from build123d import *

# Parameters (mm, degrees)
SKETCH1_W                  = 44.45
SKETCH1_H                  = 60
CUT_EXTRUDE1_START         = -50
CUT_EXTRUDE1_DEPTH         = 50
M4X0_7_TAPPED_HOLE1_D      = 3.3
M4X0_7_TAPPED_HOLE1_DEPTH  = 10
M4X0_7_TAPPED_HOLE1_TIP    = 0.991420021
M3X0_5_TAPPED_HOLE1_REACH  = 117.544
M3X0_5_TAPPED_HOLE1_BORE_R = 1.25
M3X0_5_TAPPED_HOLE2_REACH  = 117.544
M3X0_5_TAPPED_HOLE2_BORE_R = 1.25


with BuildPart() as part:
    # Sketch1 → Revolve1 (revolve)
    with BuildSketch(Plane.XZ, mode=Mode.PRIVATE) as revolve1_sk:
        with Locations((22.225, 30)):
            Rectangle(SKETCH1_W, SKETCH1_H)
    revolve(revolve1_sk.sketch.rotate(Axis((0, 0, 60), (0, 0, -1)), 180), axis=Axis((0, 0, 60), (0, 0, -1)))

    # Sketch2 → Cut-Extrude1 (cut)
    with BuildSketch(Plane(origin=(0, 0, 0), x_dir=(-1, 0, 0), z_dir=(0, 0, -1)).offset(CUT_EXTRUDE1_START)):
        with BuildLine():
            Line((43.7241638, 8), (43.7241638, -8))
            ThreePointArc((43.7241638, -8), (44.45, 0), (43.7241638, 8))
        make_face()
    extrude(amount=CUT_EXTRUDE1_DEPTH, mode=Mode.SUBTRACT)

    # Sketch3 → Cut-Revolve1 (revolve, cut)
    with BuildSketch(Plane.XZ, mode=Mode.PRIVATE) as cut_revolve1_sk:
        Polygon((37.5, 60), (0, 60), (0, 0), (37.5, 0), (37.5, 20.5), (32, 20.5), (32, 39.5), (37.5, 39.5), align=None)
    revolve(cut_revolve1_sk.sketch.rotate(Axis((0, 0, 60), (0, 0, -1)), 180), axis=Axis((0, 0, 60), (0, 0, -1)), mode=Mode.SUBTRACT)

    # M4x0.7 Tapped Hole1
    with Locations(Plane.XY.offset(60)):
        with Locations((28.991378029, 28.991378029), (0, 41), (-28.991378029, 28.991378029), (-41, 0), (-28.991378029, -28.991378029), (0, -41), (28.991378029, -28.991378029), (41, 0)):
            Hole(M4X0_7_TAPPED_HOLE1_D / 2, depth=M4X0_7_TAPPED_HOLE1_DEPTH)
            with Locations((0, 0, -(M4X0_7_TAPPED_HOLE1_DEPTH + M4X0_7_TAPPED_HOLE1_TIP / 2))):  # 118° drill point
                Cone(0, M4X0_7_TAPPED_HOLE1_D / 2, M4X0_7_TAPPED_HOLE1_TIP, mode=Mode.SUBTRACT)

    # M3x0.5 Tapped Hole1 bore → M3x0.5 Tapped Hole1 (cut, up to next)
    with BuildSketch(Plane.ZY.offset(43.7241638), mode=Mode.PRIVATE) as m3x0_5_tapped_hole1_sk1:
        with Locations((15.584748033, 5.15)):
            Circle(M3X0_5_TAPPED_HOLE1_BORE_R)
    m3x0_5_tapped_hole1_tool1 = extrude(m3x0_5_tapped_hole1_sk1.sketch, amount=-M3X0_5_TAPPED_HOLE1_REACH, mode=Mode.PRIVATE) & part.part
    add(m3x0_5_tapped_hole1_tool1.solids().sort_by_distance((-43.724164, 5.15, 15.584748))[0], mode=Mode.SUBTRACT)

    # M3x0.5 Tapped Hole2 bore → M3x0.5 Tapped Hole2 (cut, up to next)
    with BuildSketch(Plane.ZY.offset(43.7241638), mode=Mode.PRIVATE) as m3x0_5_tapped_hole2_sk1:
        with Locations((37.834748033, -5.05)):
            Circle(M3X0_5_TAPPED_HOLE2_BORE_R)
    m3x0_5_tapped_hole2_tool1 = extrude(m3x0_5_tapped_hole2_sk1.sketch, amount=-M3X0_5_TAPPED_HOLE2_REACH, mode=Mode.PRIVATE) & part.part
    add(m3x0_5_tapped_hole2_tool1.solids().sort_by_distance((-43.724164, -5.05, 37.834748))[0], mode=Mode.SUBTRACT)


solid = part.part
CAD build for the part. Positions are in the model's coordinates, mm. A direction names the side the tool comes from. Give positions to 0.01 mm unless a question says otherwise; leave off trailing zeros. Write each loop counter-clockwise with the first axis right and the second up, starting at its lowest first coordinate (ties: lowest second). Pieces come first, ordered by that corner, then holes. Notation, with made-up numbers: (68.25, -21.75) -> (87.25, -21.75) arc R21 cw to (87.25, -13.75) -> close; hole circle Ø1 at (40.25, 67.5). An arc over 180 degrees is marked (long way). Return JSON: item names as keys, results as strings.
Item 1: Band-saw the part on C-C (z = 54). Give the number of separate pieces and of enclosed holes in the cut face, then the cut area to 3 significant figures.
Answer below:
{"separate pieces": "1", "enclosed holes": "9", "area": "1,720 mm2"}
Item 2: Two-plate mould, pull along X, no slides. Class faces 5 (the cylindrical face through (-41.061, -17.025, 30.42)), 6 (the flat face through (28, 17, 39.5)), 7 (the flat face through (-32, -20, 0)): +X half, -X half, draft (parallel to the pull), parting line (faces both ways), or undercut.
Answer below:
{"face 5": "parting line", "face 6": "undercut", "face 7": "draft"}
Item 3: Tool access for faces 1 (the cylindrical face through (-37.635, -4.995, 36.586)), 2 (the cylindrical face through (42.65, 0.07, 54.93)), 3 (the flat face through (-43.724, 0, 25)), 4 (the cylindrical face through (-17.3, -33.27, 10.39)): list every direction of +Z, -Z, +X, -X, +Y, -Y with a clear straight run to the whole face (end or side of a thin tool).
Answer below:
{"face 1": "-X", "face 2": "+Z", "face 3": "-Z, -X, +Y, -Y", "face 4": "-Z"}
Item 4: Drop flat-ended pins along their axis: pin 1 (4 mm diameter, centred on x = 26.5, z = 23, fed in from +Y); pin 2 (2 mm diameter, centred on y = -5.05, z = 37.83, fed in from +X); pin 3 (12 mm diameter, centred on y = 10, z = 30, fed in from -X). Give the stop position or say it passes through.
Answer below:
{"pin 1": "stops at y = 37.09", "pin 2": "stops at x = 44.27", "pin 3": "stops at x = -43.72"}
Item 5: Band-saw the part on B-B (y = 5.15). List the corners of the cut face in (x, z), then the cut area to 3 significant figures.
Answer below:
{"outline": "(-44.15, 50) -> (-43.72, 50) -> (-43.72, 16.83) -> (-37.14, 16.83) -> (-37.14, 20.5) -> (-31.58, 20.5) -> (-31.58, 39.5) -> (-37.14, 39.5) -> (-37.14, 60) -> (-44.15, 60) -> close; (-43.72, 0) -> (-37.14, 0) -> (-37.14, 14.33) -> (-43.72, 14.33) -> close; (31.58, 20.5) -> (37.14, 20.5) -> (37.14, 0) -> (44.15, 0) -> (44.15, 60) -> (37.14, 60) -> (37.14, 39.5) -> (31.58, 39.5) -> close", "area": "1,010 mm2"}
Item 6: Band-saw the part on A-A (x = -3). List the corners of the cut face in (y, z).
Answer below:
{"outline": "(-44.35, 0) -> (-37.38, 0) -> (-37.38, 20.5) -> (-31.86, 20.5) -> (-31.86, 39.5) -> (-37.38, 39.5) -> (-37.38, 60) -> (-44.35, 60) -> close; (31.86, 20.5) -> (37.38, 20.5) -> (37.38, 0) -> (44.35, 0) -> (44.35, 60) -> (37.38, 60) -> (37.38, 39.5) -> (31.86, 39.5) -> close"}
Item 7: Band-saw the part on D-D (y = -23). List the corners of the cut face in (x, z).
Answer below:
{"outline": "(-38.04, 0) -> (-29.62, 0) -> (-29.62, 20.5) -> (-22.25, 20.5) -> (-22.25, 39.5) -> (-29.62, 39.5) -> (-29.62, 60) -> (-38.04, 60) -> close; (22.25, 20.5) -> (29.62, 20.5) -> (29.62, 0) -> (38.04, 0) -> (38.04, 60) -> (29.62, 60) -> (29.62, 39.5) -> (22.25, 39.5) -> close"}
Item 8: Drill centre lines: probe 1 along X at (y, z) = (-27.5, 50.5); probe 2 along Y at (x, z) = (0, 25); probe 3 along X at (y, z) = (-15, 33.5). Where is each one in solid material? Low to high.
Answer below:
{"probe 1": "x = -34.92 to -29.7, -28.29 to -25.5, 25.5 to 28.29, 29.7 to 34.92", "probe 2": "y = -44.45 to -32, 32 to 44.45", "probe 3": "x = -41.84 to -28.27, 28.27 to 41.84"}
